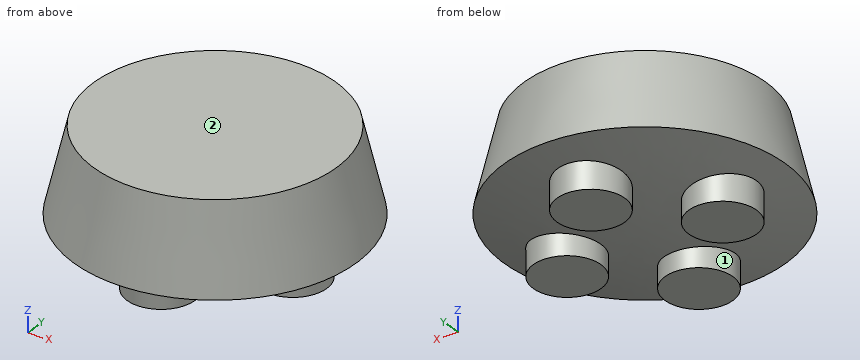
from build123d import *

# Parameters (mm, degrees)
CABLES_SKETCH_R = 35
CABLES_DEPTH    = 35


with BuildPart() as part:
    # Big Plug Sketch → Big Plug (revolve)
    with BuildSketch(Plane(origin=(0, 0, 0), x_dir=(0, 0, -1), z_dir=(1, 0, 0))):
        with BuildLine():
            Line((531.601551916, 125), (531.601551916, 0))
            Line((531.601551916, 0), (635, 0))
            ThreePointArc((635, 0), (630.771254316, 73.161634266), (618.141339438, 145.348837209))
            Line((618.141339438, 145.348837209), (531.601551916, 125))
        make_face()
    revolve(axis=Axis((0, 0, 0), (0, 0, -1)))

    # Cables Sketch → Cables (add)
    with BuildSketch(Plane.XY.offset(-618.141339438)):
        with Locations((0, 80)):
            Circle(CABLES_SKETCH_R)
        with Locations((80, 0)):
            Circle(CABLES_SKETCH_R)
        with Locations((0, -80)):
            Circle(CABLES_SKETCH_R)
        with Locations((-80, 0)):
            Circle(CABLES_SKETCH_R)
    extrude(amount=-CABLES_DEPTH)


solid = part.part
Work out the finished part from the listing and answer in its coordinate system (mm). Face numbers are marked on the shaded views. A direction names the side the tool comes from. Round coordinates to 2 decimals unless told otherwise and drop trailing zeros. Order: outer loops, then holes, each group sorted by start corner. A loop starts at its lowest first (then second) coordinate and runs counter-clockwise, first axis right, second up. Notation, with made-up numbers: M -17,54.5 L 18,54.5 A15 ccw 18,80.5 Z; hole C -27,82 d7. An arc over 180 degrees is marked long. One line per item, written item: value.
Q1. For the marked faces 1 and 2, determine the directions among +Z, -Z, +X, -X, +Y, -Y from which every point of the face is accessible in a straight line to the end or side of a thin tool.
Derived:
face 1: -Z
face 2: +Z, +X, -X, +Y, -Y
Q2. Straight lines are drawn through the part: line 1 (Y direction, x = 33, z = -583); line 2 (X direction, y = 127.5, z = -616); line 3 (X direction, y = -35.5, z = -570.5). For each, find the intervals that lie inside material, in ascending order.
Derived:
line 1: -133.05 to 133.05
line 2: -68.73 to 68.73
line 3: -129.36 to 129.36
Q3. Find section B-B on x = 0. Write down the section's boundary in (y, z), then the cut area to 3 significant figures.
Derived:
outline: M -145.35,-618.14 A635 ccw -115,-624.5 L -115,-653.14 L -45,-653.14 L -45,-633.4 A635 ccw 45,-633.4 L 45,-653.14 L 115,-653.14 L 115,-624.5 A635 ccw 145.35,-618.14 L 125,-531.6 L -125,-531.6 Z
area: 30,000 mm²
Q4. Flat-ended cylindrical pins translate along their axes: pin 1 (1 mm diameter, centred on x = -97, z = -567.5, fed in from +Y); pin 2 (6 mm diameter, centred on x = -47, y = -97.5, fed in from -Z); pin 3 (4 mm diameter, centred on x = -113, z = -638, fed in from +Y). Find the tip coordinate at first contact, or state that the pin passes through.
Derived:
pin 1: y = 92.19
pin 2: z = -626.22
pin 3: y = 16.25
Q5. Find section A-A on z = -644.5. Write down the section's boundary in (x, y), then the cut area to 3 significant figures.
Derived:
outline: C -80,0 d70; C 0,-80 d70; C 0,80 d70; C 80,0 d70
area: 15,400 mm²
Q6. Find section D-D on z = -573.5. Write down the section's boundary in (x, y).
Derived:
outline: C 0,0 d269.7
